```python
from build123d import *

# Parameters (mm, degrees)
F0_W        = 50
F0_H        = 30
F1_DEPTH    = 3.5
F2_R        = 2
F3_W        = 50
F3_H        = 3.5
F4_DEPTH    = 30
F5_T1_DEPTH = 60


# Not quite as in the source:
# - a fillet or chamfer that OpenCascade refuses, or shapes differently, is made with other operations: its cross-section is extruded or revolved along the edge and cut away or added


with BuildPart() as f1:
    # F0 (on Top) → F1 (new body)
    with BuildSketch(Plane.XY):
        Rectangle(F0_W, F0_H)
    extrude(amount=F1_DEPTH)

    # F2
    f2_edges = [f1.edges().sort_by_distance(p)[0] for p in [
        (0, 15, 3.5),
        (0, -15, 3.5),
    ]]
    fillet(f2_edges, radius=F2_R)

    # F3 (on face) → F4 (join)
    with BuildSketch(Plane.XY.offset(3.5)):
        Rectangle(F3_W, F3_H)
    extrude(amount=F4_DEPTH)

    # F5: fillet of radius 2 on 2 edges, made by hand

    # F5_s2 → F5_t1 (cut)
    with BuildSketch(Plane.YZ.offset(-30)):
        with BuildLine():
            ThreePointArc((-1.75, 31.5), (-1.1642135624, 32.9142135624), (0.25, 33.5))
            Line((0.25, 33.5), (-1.75, 33.5))
            Line((-1.75, 33.5), (-1.75, 31.5))
        make_face()
        with BuildLine():
            ThreePointArc((1.75, 31.5), (1.1642135624, 32.9142135624), (-0.25, 33.5))
            Line((-0.25, 33.5), (1.75, 33.5))
            Line((1.75, 33.5), (1.75, 31.5))
        make_face()
    extrude(amount=F5_T1_DEPTH, mode=Mode.SUBTRACT)


solid = f1.part
```
Part model, mm, in its own coordinate system. A direction names the side the tool comes from. Round coordinates to 2 decimals unless told otherwise and drop trailing zeros. Loops run counter-clockwise (first coordinate to the right, second up) from the corner with the lowest first, then second, coordinate; pieces in that order, holes last. Notation, with made-up numbers: (77, 15.5) -> (102, 15.5) arc R21 cw to (102, 25.5) -> close; hole circle Ø6 at (16, 12.25). An arc over 180 degrees is marked (long way). Use CSV: the item, a comma, the result in double quotes. Start each with the question number.
1) Which spindle directions (+Z, -Z, +X, -X, +Y, -Y) get a long thin tool onto all of the face, cutting with end or side? Do faces 1 (the flat face through (0, 7, 3.5)), 2 (the flat face through (0, 15, 1)), 3 (the flat face through (0, -1.75, 17)). Say none if no direction does.
2) Cut at B-B, the plane y = -8.75. Write the cut outline in (x, z), plus the area to 3 significant figures.
3) Cut at C-C, the plane z = 15. Write the cut outline in (x, y), plus the area to 3 significant figures.
4) Drop flat-ended pins along their axis: P1, Ø10, axis at x = -19, z = 23.5, coming from the +Y side; P2, Ø12, axis at x = -13, z = 15, coming from the -Y side; P3, Ø3.5, axis at x = -4, y = -8, coming from the +Z side. Give the stop position or say it passes through.
5) Wall check: L1, parallel to Z at x = 16.5, y = -13; L2, parallel to Y at x = 5.5, z = 6.5; L3, parallel to Y at x = 15, z = 2. Give the ranges that are in metal, low to high. Write a range as [from, to].
6) Cut at A-A, the plane x = 6. Write the cut outline in (y, z).
Determined:
1,face 1,"+Z, +X, -X, +Y"
1,face 2,"+Z, -Z, +X, -X, +Y"
1,face 3,"+Z, +X, -X, -Y"
2,outline,"(-25, 0) -> (25, 0) -> (25, 3.5) -> (-25, 3.5) -> close"
2,area,"175 mm2"
3,outline,"(-25, -1.75) -> (25, -1.75) -> (25, 1.75) -> (-25, 1.75) -> close"
3,area,"175 mm2"
4,P1,"stops at y = 1.75"
4,P2,"stops at y = -1.75"
4,P3,"stops at z = 3.5"
5,L1,"z = [0, 3.5]"
5,L2,"y = [-1.75, 1.75]"
5,L3,"y = [-14.94, 14.94]"
6,outline,"(-15, 0) -> (15, 0) -> (15, 1.5) arc R2 ccw to (13, 3.5) -> (1.75, 3.5) -> (1.75, 31.5) arc R2 ccw to (0, 33.48) arc R2 ccw to (-1.75, 31.5) -> (-1.75, 3.5) -> (-13, 3.5) arc R2 ccw to (-15, 1.5) -> close"
